Build history of the part. All positions in model axes, mm. Round coordinates to 2 decimals unless told otherwise and drop trailing zeros. Loops run counter-clockwise (first coordinate to the right, second up) from the corner with the lowest first, then second, coordinate; pieces in that order, holes last. Notation, with made-up numbers: (25.5, 85.25) - (83.5, 85.25) arc R19 ccw to (83.5, 89.25) - close; hole circle Ø9 at (68, -7.5). An arc over 180 degrees is marked (long way). Answer as CSV lines item,"result". Start each with the question number.
```python
from build123d import *

# Parameters (mm, degrees)
SKIZZE1_W                       = 80
SKIZZE1_H                       = 65
SKIZZE1_R                       = 11
SKIZZE1_R_2                     = 4.25
AUFSATZ_LINEAR_AUSTRAGEN1_DEPTH = 4
VERRUNDUNG1_R                   = 8


with BuildPart() as part:
    # Skizze1 → Aufsatz-Linear austragen1 (new, symmetric)
    with BuildSketch(Plane.XY):
        with Locations((0, -7.5)):
            Rectangle(SKIZZE1_W, SKIZZE1_H)
        Circle(SKIZZE1_R, mode=Mode.SUBTRACT)
        with Locations((-30, -30)):
            Circle(SKIZZE1_R_2, mode=Mode.SUBTRACT)
        with Locations((30, -30)):
            Circle(SKIZZE1_R_2, mode=Mode.SUBTRACT)
    extrude(amount=AUFSATZ_LINEAR_AUSTRAGEN1_DEPTH, both=True)

    # Verrundung1
    verrundung1_edges = [part.edges().sort_by_distance(p)[0] for p in [
        (-40, 25, 0),
        (40, 25, 0),
        (40, -40, 0),
        (-40, -40, 0),
    ]]
    fillet(verrundung1_edges, radius=VERRUNDUNG1_R)


solid = part.part
```
Q1. Band-saw the part on C-C, the plane x = 0. List the corners of the cut face in (y, z), then the cut area to 3 significant figures.
Q2. Band-saw the part on D-D, the plane y = -30. List the corners of the cut face in (x, z), then the cut area to 3 significant figures.
Q3. Band-saw the part on B-B, the plane z = -0.75. List the corners of the cut face in (x, y).
Q4. Wall check: probe 1 along Y at (x, z) = (30, -2); probe 2 along X at (y, z) = (-28.5, 1.5); probe 3 along X at (y, z) = (-33.5, 1.75). Give the ranges that are in metal, low to high. Write a range as [from, to].
Q5. Pin check, flat tip, straight feed: pin 1 Ø5 at (x, y) = (-30, -30) entering from +Z. Stop position of the tip, or through.
Q6. Two-plate mould, pull along X, no slides. Class faces 1 (the cylindrical face through (25.754, -29.813, -0.056)), 2 (the flat face through (40, -8, 0)), 3 (the flat face through (0, -40, 0)), 4 (the cylindrical face through (-37.719, 22.594, -0.056)): released by +X, released by -X, zero draft, split by the parting line, or undercut.
Q7. Band-saw the part on A-A, the plane y = 0. List the corners of the cut face in (x, z), then the cut area to 3 significant figures.
Reported:
1,outline,"(-40, -4) - (-11, -4) - (-11, 4) - (-40, 4) - close; (11, -4) - (25, -4) - (25, 4) - (11, 4) - close"
1,area,"344 mm2"
2,outline,"(-40, -4) - (-34.25, -4) - (-34.25, 4) - (-40, 4) - close; (-25.75, -4) - (25.75, -4) - (25.75, 4) - (-25.75, 4) - close; (34.25, -4) - (40, -4) - (40, 4) - (34.25, 4) - close"
2,area,"504 mm2"
3,outline,"(-40, -32) arc R8 ccw to (-32, -40) - (32, -40) arc R8 ccw to (40, -32) - (40, 17) arc R8 ccw to (32, 25) - (-32, 25) arc R8 ccw to (-40, 17) - close; hole circle Ø8.5 at (-30, -30); hole circle Ø22 at (0, 0); hole circle Ø8.5 at (30, -30)"
4,probe 1,"y = [-40, -34.25], [-25.75, 25]"
4,probe 2,"x = [-40, -33.98], [-26.02, 26.02], [33.98, 40]"
4,probe 3,"x = [-39.86, -32.41], [-27.59, 27.59], [32.41, 39.86]"
5,pin 1,"passes through"
6,face 1,"undercut"
6,face 2,"released by +X"
6,face 3,"zero draft"
6,face 4,"released by -X"
7,outline,"(-40, -4) - (-11, -4) - (-11, 4) - (-40, 4) - close; (11, -4) - (40, -4) - (40, 4) - (11, 4) - close"
7,area,"464 mm2"
